The listing builds one solid part. Answer for the finished solid, in the listing's coordinates (mm). A direction names the side the tool comes from. Give positions to 0.01 mm unless a question says otherwise; leave off trailing zeros. Write each loop counter-clockwise with the first axis right and the second up, starting at its lowest first coordinate (ties: lowest second). Pieces come first, ordered by that corner, then holes. Notation, with made-up numbers: (58.25, -13) -> (73.25, -13) arc R8 cw to (73.25, -1) -> close; hole circle Ø2 at (-3, 54). An arc over 180 degrees is marked (long way). Put each result on its own line as item: value. Start each with the question number.
1) A cutting plane is placed at C-C (z = -12.5). Write down the section's boundary in (x, y), then the cut area to 3 significant figures.
2) Flat-ended cylindrical pins translate along their axes: pin 1 Ø1.5 at (y, z) = (35.5, 11.5) entering from -X; pin 2 Ø1.1 at (x, z) = (-2, -13.5) entering from +Y; pin 3 Ø3 at (x, y) = (-5.5, -30.5) entering from -Z; pin 4 Ø6 at (x, y) = (-3.5, 56.5) entering from -Z. Find the tip coordinate at first contact, or state that the pin passes through.
3) For a pull along X with two mould halves and no side action, classify faces 4 (the cylindrical face through (4.506, 1.05, 14.307)), 5 (the flat face through (0, 20, 13)), 6 (the flat face through (7, 47, 7)) as released by +X, released by -X, zero draft, split by the parting line, or undercut.
4) A cutting plane is placed at D-D (y = -10). Write down the section's boundary in (x, z), then the cut area to 3 significant figures.
5) A cutting plane is placed at B-B (y = 51). Write down the section's boundary in (x, z), then the cut area to 3 significant figures.
6) A cutting plane is placed at A-A (x = 0). Write down the section's boundary in (y, z).
7) For faces 1 (the flat face through (-7, 48, 7)), 2 (the flat face through (-10, -33, 7)), 3 (the flat face through (3.5, -49, 12)), determine the directions among +Z, -Z, +X, -X, +Y, -Y from which every point of the face is accessible in a straight line to the end or side of a thin tool.
8) Find the intervals of material crossed by line 1 along Y through (x, z) = (-7.5, 10); line 2 along X through (y, z) = (-55, 0); line 3 along Y through (x, z) = (12, -1.75), in increasing order. Write a range as from..to.
from build123d import *

# Parameters (mm, degrees)
SKETCH1_R                = 15
BOSS_EXTRUDE1_DEPTH      = 75
CUT_EXTRUDE1_DEPTH       = 52
CUT_EXTRUDE2_DEPTH       = 3.5
SKETCH9_R                = 10
CUT_EXTRUDE12_DEPTH      = 70
SKETCH17_W               = 7
SKETCH17_H               = 12
CUT_EXTRUDE19_DEPTH      = 15
SKETCH19_W               = 7
SKETCH19_H               = 12
CUT_EXTRUDE20_DEPTH      = 15
SKETCH20_R               = 7.5
CUT_EXTRUDE21_DEPTH      = 40
CUT_EXTRUDE25_DEPTH      = 152.492574075
CUT_EXTRUDE25_DEPTH_BACK = 55
SKETCH21_W               = 20
SKETCH21_H               = 7.639320226
CUT_EXTRUDE27_DEPTH      = 81.841883926
CUT_EXTRUDE27_DEPTH_BACK = 81.841883926


with BuildPart() as part:
    # Sketch1 → Boss-Extrude1 (new, symmetric)
    with BuildSketch(Plane(origin=(0, 0, 0), x_dir=(1, 0, 0), z_dir=(0, 1, 0))):
        with Locations(Location((0, 0, 0), (0, 0, 270))):
            Circle(SKETCH1_R)
    extrude(amount=BOSS_EXTRUDE1_DEPTH, both=True)

    # Sketch2 → Cut-Extrude1 (cut)
    with BuildSketch(Plane.XZ.offset(75)):
        with BuildLine():
            Line((3.5, 15), (3.5, -15))
            ThreePointArc((3.5, -15), (0, -18.5), (-3.5, -15))
            Line((-3.5, -15), (-3.5, 15))
            ThreePointArc((-3.5, 15), (0, 18.5), (3.5, 15))
        make_face()
    extrude(amount=-CUT_EXTRUDE1_DEPTH, mode=Mode.SUBTRACT)

    # Sketch3 → Cut-Extrude2 (cut, symmetric)
    with BuildSketch(Plane(origin=(0, -26.5, 0), x_dir=(1, 0, 0), z_dir=(0, 1, 0))):
        Polygon((-14.980069936, 0), (-15.328117643, -9.993941304), (-0.348047707, -16.993941304), (0, -7), align=None)
        Polygon((15, 0), (0, 7), (0.348047707, 16.993941304), (15.348047707, 9.993941304), align=None)
    extrude(amount=CUT_EXTRUDE2_DEPTH, both=True, mode=Mode.SUBTRACT)

    # Sketch9 → Cut-Extrude12 (cut)
    with BuildSketch(Plane.XZ.offset(75)):
        with Locations(Location((0, 0, 0), (0, 0, 270))):
            Circle(SKETCH9_R)
    extrude(amount=-CUT_EXTRUDE12_DEPTH, mode=Mode.SUBTRACT)

    # Sketch17 → Cut-Extrude19 (cut)
    with BuildSketch(Plane(origin=(15, 0, 0), x_dir=(0, 0, -1), z_dir=(1, 0, 0))):
        with Locations((3.5, -29)):
            Rectangle(SKETCH17_W, SKETCH17_H)
    extrude(amount=-CUT_EXTRUDE19_DEPTH, mode=Mode.SUBTRACT)

    # Sketch19 → Cut-Extrude20 (cut)
    with BuildSketch(Plane.ZY.offset(15)):
        with Locations((3.5, -29)):
            Rectangle(SKETCH19_W, SKETCH19_H)
    extrude(amount=-CUT_EXTRUDE20_DEPTH, mode=Mode.SUBTRACT)

    # Sketch20 → Cut-Extrude21 (cut)
    with BuildSketch(Plane(origin=(0, 75, 0), x_dir=(1, 0, 0), z_dir=(0, 1, 0))):
        with Locations(Location((0, 0, 0), (0, 0, 270))):
            Circle(SKETCH20_R)
    extrude(amount=-CUT_EXTRUDE21_DEPTH, mode=Mode.SUBTRACT)

    # Sketch21 → Cut-Extrude25 (cut, two sides: drawn at the far end of the back side and taken through both)
    with BuildSketch(Plane(origin=(0, 75, 0), x_dir=(1, 0, 0), z_dir=(0, 1, 0)).offset(-CUT_EXTRUDE25_DEPTH_BACK)):
        with Locations((0, 15)):
            Rectangle(SKETCH21_W, SKETCH21_H)
        with Locations((0, -15)):
            Rectangle(SKETCH21_W, SKETCH21_H)
    extrude(amount=CUT_EXTRUDE25_DEPTH + CUT_EXTRUDE25_DEPTH_BACK, mode=Mode.SUBTRACT)

    # Sketch23 → Cut-Extrude27 (cut, two sides: drawn at the far end of the back side and taken through both)
    with BuildSketch(Plane(origin=(0, 0, -11.180339887), x_dir=(-1, 0, 0), z_dir=(0, 0, -1)).offset(-CUT_EXTRUDE27_DEPTH_BACK)):
        with BuildLine():
            Line((7, 55), (7, 40))
            ThreePointArc((7, 40), (0, 33), (-7, 40))
            Line((-7, 40), (-7, 55))
            ThreePointArc((-7, 55), (0, 62), (7, 55))
        make_face()
    extrude(amount=CUT_EXTRUDE27_DEPTH + CUT_EXTRUDE27_DEPTH_BACK, mode=Mode.SUBTRACT)


solid = part.part
Reply:
1. outline: (-8.29, -75) -> (-3.5, -75) -> (-3.5, -23) -> (8.29, -23) -> (8.29, 20) -> (-8.29, 20) -> close; (3.5, -75) -> (8.29, -75) -> (8.29, -30) -> (3.5, -30) -> close
1. area: 1,180 mm2
2. pin 1: stops at x = -10.46
2. pin 2: stops at y = 20
2. pin 3: stops at z = -14.46
2. pin 4: passes through
3. face 4: split by the parting line
3. face 5: zero draft
3. face 6: undercut
4. outline: circle Ø30 at (0, 0); hole circle Ø20 at (0, 0)
4. area: 393 mm2
5. outline: (-10, -11.18) -> (-7, -11.18) -> (-7, -2.69) arc R7.5 cw to (-7, 2.69) -> (-7, 11.18) -> (-10, 11.18) arc R15 ccw to start; (7, -11.18) -> (10, -11.18) arc R15 ccw to (10, 11.18) -> (7, 11.18) -> (7, 2.69) arc R7.5 cw to (7, -2.69) -> close
5. area: 285 mm2
6. outline: (-23, -15) -> (20, -15) -> (20, -11.18) -> (33, -11.18) -> (33, 11.18) -> (20, 11.18) -> (20, 15) -> (-23, 15) -> (-23, 10) -> (-5, 10) -> (-5, -10) -> (-23, -10) -> close; (62, -11.18) -> (75, -11.18) -> (75, -7.5) -> (62, -7.5) -> close; (62, 7.5) -> (75, 7.5) -> (75, 11.18) -> (62, 11.18) -> close
7. face 1: +Z, -Z
7. face 2: -X
7. face 3: +Z, -Z, -Y
8. line 1: y = -75..-30, -23..75
8. line 2: x = -15..-10, 10..15
8. line 3: y = -75..-35, -23..75
